Design review of the part built by this model. Coordinates are the model's own, in mm. A direction names the side the tool comes from. Coordinates: 2 decimals unless noted, no trailing zeros. Loops run counter-clockwise (first coordinate to the right, second up) from the corner with the lowest first, then second, coordinate; pieces in that order, holes last.
Q1. Add section A-A on x = 0. Give the boundary of the cut face in (y, z).
Q2. Draft analysis for pull direction Z (two halves, no side actions). For faces 1 (the face through (0, 2, -14)), 2 (the face through (0.672, 2.535, -9.554)), 3 (the face through (-7.5, 11, -4)), state which applies: released by +Z, released by -Z, zero draft, split by the parting line, or undercut.
Q3. For P1, Ø4.5, axis at x = -2.5, z = -8.5, coming from the +Y side, flat-tipped, find the tip position at first contact; note if it passes through.
Q4. Wall thickness on probe 1 along Z at (x, y) = (0, 2); probe 2 along X at (y, z) = (3.7, -8.5); probe 3 along Z at (x, y) = (-6, 23.25): over which ranges is each line inside the solid? List them lowest first.
Q5. Add section B-B on z = -8.5. Give the boundary of the cut face in (x, y), and give its area (3 significant figures).
Q6. Add section D-D on x = -5.5. Give the boundary of the cut face in (y, z), and give its area (3 significant figures).
Q7. Machinability: for faces 4 (the face through (0, 17, -5)), 5 (the face through (0, 30, -3)), which of the approach directions +Z, -Z, +X, -X, +Y, -Y give a long, thin tool a straight path to every point of the face, cutting with its end or side? Answer none if there is none.
Q8. Add section C-C on y = 4.25. Give the boundary of the cut face in (x, z).
Autodesk Inventor part; units mm, degrees
ref_plane "YZ Plane" through (0, 0, 0) normal (1, 0, 0) x (0, 1, 0)
ref_plane "XZ Plane" through (0, 0, 0) normal (0, 1, 0) x (-1, 0, 0)
ref_plane "XY Plane" through (0, 0, 0) normal (0, 0, 1) x (1, 0, 0)
sketch "Sketch1" plane through (0, 0, 0) normal (1, 0, 0) x (0, 1, 0)
  line L0 (30, 0) -> (0, 0)
  line L1 (0, 0) -> (0, -14)
  line L2 (0, -14) -> (5, -14)
  line L3 (5, -14) -> (5, -5)
  line L4 (5, -5) -> (30, -5)
  line L5 (30, -5) -> (30, 0)
  dimension "d0" = 5
  dimension "d1" = 14
  dimension "d2" = 5
  dimension "d3" = 30
extrude "Extrusion1" add sketch "Sketch1" against normal mid plane 15
sketch "Sketch2" plane through (-7.5, 5, -14) normal (0, 1, 0) x (1, 0, 0)
  circle A0 centre (7.5, -5.5) radius 1.25
  line L0 (0, 0) -> (15, 0)
  line L1 (0, -14) -> (15, -14)
  line L2 (0, -9) -> (15, -9)
  point P0 (7.5, -14)
  point P1 (7.5, -14)
  dimension "d6" = 2.5
  dimension "d10" = 3.5
extrude "Extrusion2" cut sketch "Sketch2" against normal through all
properties part number "battery_fix_board"
Entries:
1. outline: (0, -14) - (5, -14) - (5, -9.75) - (0, -9.75) - close; (0, -7.25) - (5, -7.25) - (5, -5) - (30, -5) - (30, 0) - (0, 0) - close
2. face 1: released by -Z
2. face 2: undercut
2. face 3: zero draft
3. P1: stops at y = 5
4. probe 1: z = -14 to -9.75, -7.25 to 0
4. probe 2: x = -7.5 to -1.25, 1.25 to 7.5
4. probe 3: z = -5 to 0
5. outline: (-7.5, 0) - (-1.25, 0) - (-1.25, 5) - (-7.5, 5) - close; (1.25, 0) - (7.5, 0) - (7.5, 5) - (1.25, 5) - close
5. area: 62.5 mm2
6. outline: (0, -14) - (5, -14) - (5, -5) - (30, -5) - (30, 0) - (0, 0) - close
6. area: 195 mm2
7. face 4: -Z, +X, -X, +Y
7. face 5: +Z, -Z, +X, -X, +Y
8. outline: (-7.5, -14) - (7.5, -14) - (7.5, 0) - (-7.5, 0) - close; hole circle Ø2.5 at (0, -8.5)
